from build123d import *

# Parameters (mm, degrees)
SKETCH_2_W                    = 4.2
SKETCH_2_H                    = 1
CUT_EXTRUDE_1_DEPTH           = 1
CUT_EXTRUDE_1_DRAFT           = -15
SKETCH_2_W_2                  = 1
SKETCH_2_H_2                  = 4.2
CUT_EXTRUDE_1_PROFILE_2_DEPTH = 1
CUT_EXTRUDE_1_PROFILE_2_DRAFT = -15
CHAMFER_1_SIZE                = 0.1


with BuildPart() as part:
    # 草图1 → 旋转1 (revolve)
    with BuildSketch(Plane.XY, mode=Mode.PRIVATE) as revolve_1_sk:
        with BuildLine():
            Line((0, 0), (1.5, 0))
            Line((1.5, 0), (1.5, 5))
            Line((1.5, 5), (2.1, 5))
            ThreePointArc((2.1, 5), (2.533998358, 5.948381153), (1.780839976, 6.669861464))
            ThreePointArc((1.780839976, 6.669861464), (0.892794357, 6.767422046), (0, 6.8))
            Line((0, 6.8), (0, 0))
        make_face()
    revolve(revolve_1_sk.sketch.rotate(Axis((0, 7.002401016, 0), (0, -1, 0)), 90), axis=Axis((0, 7.002401016, 0), (0, -1, 0)))


with BuildPart() as cut_extrude_1_tool:
    # 草图2 → 切除-拉伸1 (with draft: the straight prism first)
    with BuildSketch(Plane(origin=(0, 6.8, 0), x_dir=(1, 0, 0), z_dir=(0, 1, 0))):
        Rectangle(SKETCH_2_W, SKETCH_2_H)
    extrude(amount=-CUT_EXTRUDE_1_DEPTH)
    # 切除-拉伸1: the draft: its side faces are tilted about the plane it starts from
    cut_extrude_1_sides = [cut_extrude_1_tool.faces().sort_by_distance(p)[0] for p in [
        (0, 6.3, 0.5),
        (2.1, 6.3, 0),
        (0, 6.3, -0.5),
        (-2.1, 6.3, 0),
    ]]
    draft(cut_extrude_1_sides, Plane(origin=(0, 6.8, 0), x_dir=(1, 0, 0), z_dir=(0, 1, 0)), CUT_EXTRUDE_1_DRAFT)


with BuildPart() as part_1:
    add(part.part)

    # 切除-拉伸1: cut by cut_extrude_1_tool
    add(cut_extrude_1_tool.part, mode=Mode.SUBTRACT)


with BuildPart() as cut_extrude_1_profile_2_tool:
    # 草图2 → 切除-拉伸1 profile 2 (with draft: the straight prism first)
    with BuildSketch(Plane(origin=(0, 6.8, 0), x_dir=(1, 0, 0), z_dir=(0, 1, 0))):
        Rectangle(SKETCH_2_W_2, SKETCH_2_H_2)
    extrude(amount=-CUT_EXTRUDE_1_PROFILE_2_DEPTH)
    # 切除-拉伸1 profile 2: the draft: its side faces are tilted about the plane it starts from
    cut_extrude_1_profile_2_sides = [cut_extrude_1_profile_2_tool.faces().sort_by_distance(p)[0] for p in [
        (0, 6.3, 2.1),
        (0.5, 6.3, 0),
        (0, 6.3, -2.1),
        (-0.5, 6.3, 0),
    ]]
    draft(cut_extrude_1_profile_2_sides, Plane(origin=(0, 6.8, 0), x_dir=(1, 0, 0), z_dir=(0, 1, 0)), CUT_EXTRUDE_1_PROFILE_2_DRAFT)


with BuildPart() as part_2:
    add(part_1.part)

    # 切除-拉伸1 profile 2: cut by cut_extrude_1_profile_2_tool
    add(cut_extrude_1_profile_2_tool.part, mode=Mode.SUBTRACT)

    # 倒角1
    chamfer_1_edges = [part_2.edges().sort_by_distance(p)[0] for p in [
        (0, 0, -1.5),
    ]]
    chamfer(chamfer_1_edges, length=CHAMFER_1_SIZE)


solid = part_2.part
Work out the finished part from the listing and answer in its coordinate system (mm). A direction names the side the tool comes from. Coordinates: 2 decimals unless noted, no trailing zeros. Write each loop counter-clockwise with the first axis right and the second up, starting at its lowest first coordinate (ties: lowest second). Pieces come first, ordered by that corner, then holes. Notation, with made-up numbers: M -17,52.25 L 19,52.25 A10 ccw 19,60.25 Z; hole C 29.5,65 d9. An arc over 180 degrees is marked long. Answer as CSV lines item,"result". Start each with the question number.
Item 1: Consider L1, parallel to Y at x = 0, z = -0.3; L2, parallel to X at y = 6, z = 1.7; L3, parallel to X at y = 5.25, z = 1.35. Determine where each line is inside the solid, lowest interval first.
Item 2: Section A-A on z = 0 is taken. Write down the section's boundary in (x, y), and give its area (3 significant figures).
Item 3: Determine the mould class of faces 3 (the face through (0, 0, 0)), 4 (the face through (-1.148, 6.297, 0.365)), 5 (the face through (1.122, 6.297, -0.365)), 6 (the face through (-0.45, 2.58, 1.43)) for opening direction X: released by +X, released by -X, zero draft, split by the parting line, or undercut.
Item 4: A tool of negligible diameter and unlimited length cuts with its end or side. For faces 1 (the face through (0.365, 6.297, 1.148)), 2 (the face through (0.9, 5, -1.4)), from which of +Z, -Z, +X, -X, +Y, -Y can it reach the whole face along a straight path? Write none if from no direction.
Item 5: Section D-D on y = 6 is taken. Write down the section's boundary in (x, z).
Item 6: Section B-B on x = 0 is taken. Write down the section's boundary in (y, z).
Item 7: Section C-C on y = 1.25 is taken. Write down the section's boundary in (x, z), and give its area (3 significant figures).
Item 8: A flat-ended cylindrical pin translates along its axis: P1, Ø2, axis at x = 2, y = 4.5, coming from the -Z side. Find the tip coordinate at first contact, or state that the pin passes through.
Checks:
1,L1,"y = 0 to 5.8"
1,L2,"x = -1.86 to -0.29, 0.29 to 1.86"
1,L3,"x = -1.96 to 1.96"
2,outline,"M -2.1,5 L -1.5,5 L -1.5,0.1 L -1.4,0 L 1.4,0 L 1.5,0.1 L 1.5,5 L 2.1,5 A0.9 ccw 2.04,6.59 L 1.83,5.8 L -1.83,5.8 L -2.04,6.59 A0.9 ccw Z"
2,area,"19.6 mm²"
3,face 3,"zero draft"
3,face 4,"undercut"
3,face 5,"undercut"
3,face 6,"split by the parting line"
4,face 1,"+Y"
4,face 2,"-Y"
5,outline,"C 0,0 d5.05; hole M -1.89,-0.29 L -0.29,-0.29 L -0.29,-1.89 L 0.29,-1.89 L 0.29,-0.29 L 1.89,-0.29 L 1.89,0.29 L 0.29,0.29 L 0.29,1.89 L -0.29,1.89 L -0.29,0.29 L -1.89,0.29 Z"
6,outline,"M 0,-1.4 L 0.1,-1.5 L 5,-1.5 L 5,-2.1 A0.9 ccw 6.59,-2.04 L 5.8,-1.83 L 5.8,1.83 L 6.59,2.04 A0.9 ccw 5,2.1 L 5,1.5 L 0.1,1.5 L 0,1.4 Z"
7,outline,"C 0,0 d3"
7,area,"7.07 mm²"
8,P1,"stops at z = -1.97"
